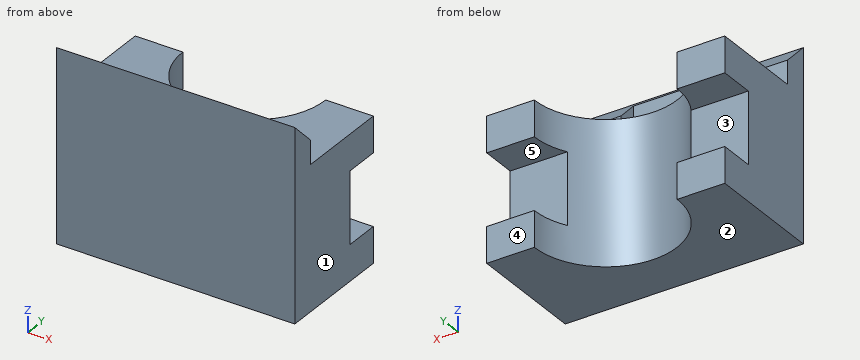
from build123d import *

# Parameters (mm, degrees)
BOSS_EXTRUDE1_DEPTH = 50
CUT_EXTRUDE1_DEPTH  = 100
SKETCH3_W           = 40
SKETCH3_H           = 8
CUT_EXTRUDE2_DEPTH  = 100


with BuildPart() as part:
    # Sketch1 → Boss-Extrude1 (new body, symmetric)
    with BuildSketch(Plane(origin=(0, 0, 0), x_dir=(0, 0, -1), z_dir=(1, 0, 0))):
        Polygon((-40, 0), (40, 0), (40, 50), (25, 50), (25, 35), (-5, 35), (-5, 50), (-20, 50), (-20, 10), (-30, 10), align=None)
    extrude(amount=BOSS_EXTRUDE1_DEPTH, both=True)

    # Sketch2 → Cut-Extrude1 (cut)
    with BuildSketch(Plane.XY.offset(20)):
        with BuildLine():
            Line((-30, 50), (30, 50))
            ThreePointArc((30, 50), (0, 20), (-30, 50))
        make_face()
    extrude(amount=-CUT_EXTRUDE1_DEPTH, mode=Mode.SUBTRACT)

    # Sketch3 → Cut-Extrude2 (cut)
    with BuildSketch(Plane.XY.offset(20)):
        with Locations((0, 6)):
            Rectangle(SKETCH3_W, SKETCH3_H)
    extrude(amount=CUT_EXTRUDE2_DEPTH, mode=Mode.SUBTRACT)


solid = part.part
Source: CAD feature listing. Evaluate the final solid. Frame: model axes, mm. Face numbers are marked on the shaded views. A direction names the side the tool comes from. Round coordinates to 2 decimals unless told otherwise and drop trailing zeros. Write each loop counter-clockwise with the first axis right and the second up, starting at its lowest first coordinate (ties: lowest second). Pieces come first, ordered by that corner, then holes. Notation, with made-up numbers: (77, -39.75) - (130, -39.75) arc R30 ccw to (130, -16.75) - close; hole circle Ø7 at (67, 9.5). An arc over 180 degrees is marked (long way). Use CSV: the item, a comma, the result in double quotes. Start each with the question number.
(1) Cut plane C-C, the plane z = -35. Return loops of the section in (x, y), and give its area (3 significant figures).
(2) First-contact query: pin 1 Ø4 at (x, z) = (22, -5.5) entering from +Y; pin 2 Ø19 at (x, z) = (32, -7) entering from +Y; pin 3 Ø6 at (x, z) = (20, -5) entering from +Y. Flat tips, straight axial feed; report the tip coordinate or a pass-through.
(3) Cut plane B-B, the plane x = 18. Return loops of the section in (y, z), and give its area (3 significant figures).
(4) Cut plane A-A, the plane y = 30. Return loops of the section in (x, z), and give its area (3 significant figures).
(5) Set-up query: the marked faces 4 and 5. Return all of +Z, -Z, +X, -X, +Y, -Y with unobstructed straight access to the full face (end or side cutting, diameter ignored); none if empty.
(6) Material intervals for probe 1 along Z at (x, y) = (36.5, 40.5); probe 2 along Z at (x, y) = (39, 21.5); probe 3 along Y at (x, z) = (12.5, 32), sorted ascending. Write a range as [from, to].
(7) Cut plane D-D, the plane y = 38. Return loops of the section in (x, z).
(8) Mould query, pull axis Z, two halves, no side actions, for the marked faces 1, 2 and 3. Classes: pulls with the +Z half, pulls with the -Z half, needs draft (parallel to the pull), parting line crosses it, or undercut.
Geometry says:
1,outline,"(-50, 0) - (50, 0) - (50, 50) - (30, 50) arc R30 cw to (-30, 50) - (-50, 50) - close"
1,area,"3,590 mm²"
2,pin 1,"y = 32"
2,pin 2,"y = 35"
2,pin 3,"y = 30.74"
3,outline,"(0, -40) - (26, -40) - (26, 20) - (2, 20) - (2, 38) - (0, 40) - close"
3,area,"1,600 mm²"
4,outline,"(-50, -40) - (-22.36, -40) - (-22.36, 20) - (-50, 20) - close; (22.36, -40) - (50, -40) - (50, 20) - (22.36, 20) - close"
4,area,"3,320 mm²"
5,face 4,"+Z, -Z, +X, -X, +Y"
5,face 5,"+X, -X, +Y"
6,probe 1,"[-40, -25], [5, 20]"
6,probe 2,"[-40, 20]"
6,probe 3,"[0, 2]"
7,outline,"(-50, -40) - (-27.5, -40) - (-27.5, -25) - (-50, -25) - close; (-50, 5) - (-27.5, 5) - (-27.5, 20) - (-50, 20) - close; (27.5, -40) - (50, -40) - (50, -25) - (27.5, -25) - close; (27.5, 5) - (50, 5) - (50, 20) - (27.5, 20) - close"
8,face 1,"needs draft"
8,face 2,"pulls with the -Z half"
8,face 3,"undercut"
